```python
from build123d import *

# Parameters (mm, degrees)
F1_DEPTH  = 5
F3_DEPTH  = 20
F6_R      = 2.4197546063
F7_DEPTH  = 25
F8_R      = 5
F9_R      = 5
F10_R     = 1
F4_R      = 2
F11_DEPTH = 10
F5_R      = 2
F12_DEPTH = 10


with BuildPart() as f1:
    # F0 (on Top) → F1 (new body)
    with BuildSketch(Plane.XY):
        Polygon((-23.4292047727, 30), (-53.4292047727, 30), (-53.4292047727, -30), (6.5707952273, -30), (6.5707952273, 0), align=None)
    extrude(amount=F1_DEPTH)

    # F2 (on face) → F3 (join)
    with BuildSketch(Plane.XY.offset(5)):
        Polygon((6.5707952273, -30), (6.5707952273, -25), (-48.4292047727, -25), (-48.4292047727, 30), (-53.4292047727, 30), (-53.4292047727, -30), align=None)
        Polygon((-28.4292047727, 30), (-28.4292047727, -5), (6.5707952273, -5), (6.5707952273, 0), (-23.4292047727, 0), (-23.4292047727, 30), align=None)
    extrude(amount=F3_DEPTH)

    # F6 (on face) → F7 (cut)
    with BuildSketch(Plane.XY.offset(5)):
        with Locations((-15.4292047727, 8)):
            Circle(F6_R)
    extrude(amount=-F7_DEPTH, mode=Mode.SUBTRACT)

    # F8
    f8_edges = [f1.edges().sort_by_distance(p)[0] for p in [
        (-23.429205, 0, 15),
    ]]
    fillet(f8_edges, radius=F8_R)

    # F9
    f9_edges = [f1.edges().sort_by_distance(p)[0] for p in [
        (-53.429205, -30, 12.5),
    ]]
    fillet(f9_edges, radius=F9_R)

    # F10
    f10_edges = [f1.edges().sort_by_distance(p)[0] for p in [
        (-20.929205, -30, 25),
        (-23.429205, 17.5, 25),
        (-53.429205, 2.5, 25),
        (-51.964739, -28.535534, 25),
        (-5.929205, 0, 25),
        (-21.964739, 1.464466, 25),
    ]]
    fillet(f10_edges, radius=F10_R)

    # F4 (on face) → F11 (cut)
    with BuildSketch(Plane.YZ.offset(-23.4292047727)):
        with Locations((15, 15)):
            Circle(F4_R)
    extrude(amount=-F11_DEPTH, mode=Mode.SUBTRACT)

    # F5 (on face) → F12 (cut)
    with BuildSketch(Plane(origin=(0, 0, 0), x_dir=(-1, 0, 0), z_dir=(0, 1, 0))):
        with Locations((8.4292047727, 15)):
            Circle(F5_R)
    extrude(amount=-F12_DEPTH, mode=Mode.SUBTRACT)


solid = f1.part
```
Check sheet for the modelled part. Datum: model origin and axes. Units: mm. A direction names the side the tool comes from. Round coordinates to 2 decimals unless told otherwise and drop trailing zeros. Order: outer loops, then holes, each group sorted by start corner. A loop starts at its lowest first (then second) coordinate and runs counter-clockwise, first axis right, second up.
1) Section check C-C (z = 15). Record the boundary of the cut face in (x, y), and give its area (3 significant figures).
2) Section check A-A (z = 10). Record the boundary of the cut face in (x, y).
3) Mould release check, pull along Z, two halves, no side actions. Record for faces 1 (the cylindrical face through (-8.169, -2.465, 16.983)), 2 (the flat face through (-12, 9, 5)), 3 (the flat face through (-11, -5, 15)), 4 (the cylindrical face through (-26, 15, 17)): +Z half, -Z half, draft (parallel to the pull), parting line (faces both ways), or undercut.
4) Scan lines: line 1 (Y direction, x = 4.5, z = 19.5); line 2 (Z direction, x = -27.25, y = 15); line 3 (X direction, y = 11, z = 11). Record each from-to range of solid material in increasing order.
5) Section check B-B (y = 14). Record the boundary of the cut face in (x, z).
6) Section check D-D (x = -40.5). Record the boundary of the cut face in (y, z), and give its area (3 significant figures).
7) Go/stop test with flat-tipped pins: pin 1 Ø10 at (y, z) = (18, 18.5) entering from +X; pin 2 Ø7.5 at (x, y) = (-15.43, 8) entering from +Z; pin 3 Ø8 at (y, z) = (-19, 8.5) entering from +X. Record where each tip stops, or that it passes through.
8) Tool access check on faces 5 (the flat face through (6.571, -19, 4)), 6 (the cylindrical face through (-21.9, 1.4, 14.6)), 7 (the flat face through (-48.429, 2, 15)). Record the directions out of +Z, -Z, +X, -X, +Y, -Y that give a thin tool (end or side, any length) a straight path to the whole face; none if there is none.
Result:
1. outline: (-53.43, -25) arc R5 ccw to (-48.43, -30) - (6.57, -30) - (6.57, -25) - (-48.43, -25) - (-48.43, 30) - (-53.43, 30) - close; (-28.43, -5) - (-10.43, -5) - (-10.43, 0) - (-18.43, 0) arc R5 cw to (-23.43, 5) - (-23.43, 13) - (-28.43, 13) - close; (-28.43, 17) - (-23.43, 17) - (-23.43, 30) - (-28.43, 30) - close; (-6.43, -5) - (6.57, -5) - (6.57, 0) - (-6.43, 0) - close
1. area: 860 mm2
2. outline: (-53.43, -25) arc R5 ccw to (-48.43, -30) - (6.57, -30) - (6.57, -25) - (-48.43, -25) - (-48.43, 30) - (-53.43, 30) - close; (-28.43, -5) - (6.57, -5) - (6.57, 0) - (-18.43, 0) arc R5 cw to (-23.43, 5) - (-23.43, 30) - (-28.43, 30) - close
3. face 1: undercut
3. face 2: +Z half
3. face 3: draft
3. face 4: undercut
4. line 1: y = -30 to -25, -5 to 0
4. line 2: z = 0 to 13, 17 to 25
4. line 3: x = -53.43 to -48.43, -28.43 to -23.43
5. outline: (-53.43, 0) - (-7.43, 0) - (-7.43, 5) - (-23.43, 5) - (-23.43, 13.27) - (-28.43, 13.27) - (-28.43, 5) - (-48.43, 5) - (-48.43, 25) - (-52.43, 25) arc R1 ccw to (-53.43, 24) - close; (-28.43, 16.73) - (-23.43, 16.73) - (-23.43, 24) arc R1 ccw to (-24.43, 25) - (-28.43, 25) - close
6. outline: (-30, 0) - (30, 0) - (30, 5) - (-25, 5) - (-25, 25) - (-29, 25) arc R1 ccw to (-30, 24) - close
6. area: 400 mm2
7. pin 1: stops at x = -23.43
7. pin 2: stops at z = 5
7. pin 3: stops at x = 6.57
8. face 5: +Z, -Z, +X, +Y, -Y
8. face 6: +Z, +X, +Y
8. face 7: +Z, +Y
